Read the model definition and answer for the solid it produces. Units are mm, in the model's axes. A direction names the side the tool comes from. Give positions to 0.01 mm unless a question says otherwise; leave off trailing zeros. Write each loop counter-clockwise with the first axis right and the second up, starting at its lowest first coordinate (ties: lowest second). Pieces come first, ordered by that corner, then holes. Notation, with made-up numbers: (62, 25) -> (85, 25) arc R3 ccw to (85, 30) -> close; hole circle Ø10 at (45.25, 55). An arc over 180 degrees is marked (long way). Write item = value, one per line.
from build123d import *

# Parameters (mm, degrees)
F0_W           = 27
F0_H           = 40
F1_DEPTH       = 32
F3_D           = 3.3
F3_CBORE_D     = 6.5
F3_CBORE_DEPTH = 10
F4_D           = 5


with BuildPart() as f1:
    # F0 (on Top) → F1 (new body)
    with BuildSketch(Plane.XY):
        with Locations((-23.3004702032, -43.8329163194)):
            Rectangle(F0_W, F0_H)
    extrude(amount=F1_DEPTH)

    # F3 (through all)
    with Locations(Plane.XY.offset(32)):
        with Locations((-33.3004702032, -33.8329163194), (-13.3004702032, -33.8329163194), (-13.3004702032, -53.8329163194), (-33.3004702032, -53.8329163194)):
            CounterBoreHole(F3_D / 2, F3_CBORE_D / 2, F3_CBORE_DEPTH)

    # F4 (through all)
    with Locations(Plane.XY.offset(32)):
        with Locations((-23.3004702032, -28.8329163194), (-23.3004702032, -58.8329163194)):
            Hole(F4_D / 2)


solid = f1.part
(1) Consider L1, parallel to Y at x = -23.5, z = 1.5; L2, parallel to X at y = -54.5, z = 6.5; L3, parallel to Y at x = -33, z = 24.5. Determine where each line is inside the solid, lowest interval first.
Checks:
L1 = -63.83 to -61.32, -56.34 to -31.32, -26.34 to -23.83
L2 = -36.8 to -34.81, -31.79 to -14.81, -11.79 to -9.8
L3 = -63.83 to -57.07, -50.6 to -37.07, -30.6 to -23.83
(2) The part is cut by section D-D on y = -30. Determine the outline of the cut face in (x, z), plus the area to 3 significant figures.
Checks:
outline = (-36.8, 0) -> (-25.51, 0) -> (-25.51, 32) -> (-36.8, 32) -> close; (-21.09, 0) -> (-9.8, 0) -> (-9.8, 32) -> (-21.09, 32) -> close
area = 723 mm²
(3) A tool of negligible diameter and unlimited length cuts with its end or side. For faces 4 (the cylindrical face through (-35.7, -31.64, 27.07)), 5 (the flat face through (-23, -44, 32)), from which of +Z, -Z, +X, -X, +Y, -Y can it reach the whole face along a straight path? Write none if from no direction.
Checks:
face_4 = +Z
face_5 = +Z, +X, -X, +Y, -Y
(4) The part is cut by section A-A on x = -33.5. Determine the outline of the cut face in (y, z).
Checks:
outline = (-63.83, 0) -> (-55.47, 0) -> (-55.47, 22) -> (-57.08, 22) -> (-57.08, 32) -> (-63.83, 32) -> close; (-52.2, 0) -> (-35.47, 0) -> (-35.47, 22) -> (-37.08, 22) -> (-37.08, 32) -> (-50.59, 32) -> (-50.59, 22) -> (-52.2, 22) -> close; (-32.2, 0) -> (-23.83, 0) -> (-23.83, 32) -> (-30.59, 32) -> (-30.59, 22) -> (-32.2, 22) -> close
(5) The part is cut by section B-B on y = -54.5. Determine the outline of the cut face in (x, z), plus the area to 3 significant figures.
Checks:
outline = (-36.8, 0) -> (-34.81, 0) -> (-34.81, 22) -> (-36.48, 22) -> (-36.48, 32) -> (-36.8, 32) -> close; (-31.79, 0) -> (-14.81, 0) -> (-14.81, 22) -> (-16.48, 22) -> (-16.48, 32) -> (-30.12, 32) -> (-30.12, 22) -> (-31.79, 22) -> close; (-11.79, 0) -> (-9.8, 0) -> (-9.8, 32) -> (-10.12, 32) -> (-10.12, 22) -> (-11.79, 22) -> close
area = 604 mm²
(6) Given P1, Ø3, axis at x = -13, y = -32.5, coming from the +Z side, flat-ended and moving along its own axis, determine where the tip first touches the part or whether it passes through.
Checks:
P1 = 22
(7) The part is cut by section C-C on z = 17. Determine the outline of the cut face in (x, y).
Checks:
outline = (-36.8, -63.83) -> (-9.8, -63.83) -> (-9.8, -23.83) -> (-36.8, -23.83) -> close; hole circle Ø3.3 at (-33.3, -53.83); hole circle Ø3.3 at (-33.3, -33.83); hole circle Ø5 at (-23.3, -58.83); hole circle Ø5 at (-23.3, -28.83); hole circle Ø3.3 at (-13.3, -53.83); hole circle Ø3.3 at (-13.3, -33.83)
(8) For a pull along X with two mould halves and no side action, classify faces 1 (the cylindrical face through (-13.72, -30.61, 27.07)), 2 (the flat face through (-23, -63.833, 16)), 3 (the flat face through (-36.8, -44, 16)) as released by +X, released by -X, zero draft, split by the parting line, or undercut.
Checks:
face_1 = undercut
face_2 = zero draft
face_3 = released by -X
